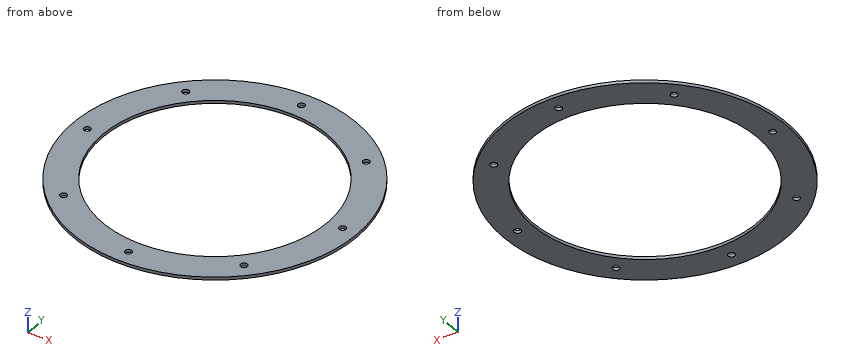
```python
from build123d import *

# Parameters (mm, degrees)
SKETCH1_R          = 192
SKETCH1_R_2        = 152
BASE_FLANGE1_DEPTH = 4
SKETCH2_R          = 4.5
CUT_EXTRUDE1_DEPTH = 10
CIRPATTERN1_COUNT  = 8


# Sheet-metal steps are written as plain solids
with BuildPart() as part:
    # Sketch1 → Base-Flange1 (new body)
    with BuildSketch(Plane.XY):
        Circle(SKETCH1_R)
        Circle(SKETCH1_R_2, mode=Mode.SUBTRACT)
    extrude(amount=-BASE_FLANGE1_DEPTH)

    # Sketch2 → Cut-Extrude1 (cut)
    with BuildSketch(Plane.XY):
        with Locations((0, 172)):
            Circle(SKETCH2_R)
    cut_extrude1 = extrude(amount=-CUT_EXTRUDE1_DEPTH, mode=Mode.SUBTRACT)

    # CirPattern1: Cut-Extrude1 ×8 about axis
    cirpattern1_axis = Axis((0, 0, 0), (0, 0, 1))
    for i in range(1, CIRPATTERN1_COUNT):
        add(cut_extrude1.rotate(cirpattern1_axis, i * 360 / CIRPATTERN1_COUNT), mode=Mode.SUBTRACT)


solid = part.part
```
Geometry check sheet. Reference: the model listing, model coordinates, mm. Coordinates: 2 decimals unless noted, no trailing zeros. Order: outer loops, then holes, each group sorted by start corner. A loop starts at its lowest first (then second) coordinate and runs counter-clockwise, first axis right, second up.
Item 1: Section check A-A (y = 38.5). Enter the section's corners in (x, z).
Item 2: Scan lines: line 1 along Y through (x, z) = (0, -2.3); line 2 along Y through (x, z) = (117.5, -2.1); line 3 along X through (y, z) = (-120.5, -2.75). Record each from-to range of solid material in increasing order.
Item 3: Section check B-B (x = 0). Enter the section's corners in (y, z), plus the area to 3 significant figures.
Item 4: Depth check by flat-ended pin: pin 1 (11.5 mm diameter, centred on x = -121.62, y = -121.62, fed in from -Z). Enter the tip coordinate at first touch or a pass-through.
Item 5: Section check C-C (z = -1.35). Count the separate pieces of the cut face and the enclosed holes in it, plus the area to 3 significant figures.
Item 6: Section check D-D (x = -101.5). Enter the section's corners in (y, z), plus the area to 3 significant figures.
Check sheet entries:
1. outline: (-188.1, -4) - (-147.04, -4) - (-147.04, 0) - (-188.1, 0) - close; (147.04, -4) - (188.1, -4) - (188.1, 0) - (147.04, 0) - close
2. line 1: y = -192 to -176.5, -167.5 to -152, 152 to 167.5, 176.5 to 192
2. line 2: y = -151.85 to -123.43, -119.82 to -96.42, 96.42 to 119.82, 123.43 to 151.85
2. line 3: x = -149.48 to -125.98, -117.26 to -92.65, 92.65 to 117.26, 125.98 to 149.48
3. outline: (-192, -4) - (-176.5, -4) - (-176.5, 0) - (-192, 0) - close; (-167.5, -4) - (-152, -4) - (-152, 0) - (-167.5, 0) - close; (152, -4) - (167.5, -4) - (167.5, 0) - (152, 0) - close; (176.5, -4) - (192, -4) - (192, 0) - (176.5, 0) - close
3. area: 248 mm2
4. pin 1: stops at z = -4
5. separate pieces: 1
5. enclosed holes: 9
5. area: 42,700 mm2
6. outline: (-162.98, -4) - (-113.14, -4) - (-113.14, 0) - (-162.98, 0) - close; (113.14, -4) - (162.98, -4) - (162.98, 0) - (113.14, 0) - close
6. area: 399 mm2
